Design review of the part built by this model. Coordinates are the model's own, in mm. Round coordinates to 2 decimals unless told otherwise and drop trailing zeros. Loops run counter-clockwise (first coordinate to the right, second up) from the corner with the lowest first, then second, coordinate; pieces in that order, holes last. Notation, with made-up numbers: (32.25, 40.5) - (53.25, 40.5) arc R6 ccw to (53.25, 51.5) - close; hole circle Ø11 at (61, 85.5). An arc over 180 degrees is marked (long way). Return JSON: item names as keys, results as strings. Group by question number.
from build123d import *

# Parameters (mm, degrees)
SKETCH1_R           = 92.075
SKETCH1_R_2         = 88.9
BOSS_EXTRUDE1_DEPTH = 38.1
SKETCH3_R           = 1.35255
CUT_EXTRUDE1_DEPTH  = 34.798
CIRPATTERN1_COUNT   = 3


with BuildPart() as part:
    # Sketch1 → Boss-Extrude1 (new, symmetric)
    with BuildSketch(Plane(origin=(0, 0, 0), x_dir=(1, 0, 0), z_dir=(0, 1, 0))):
        with Locations(Location((0, 0, 0), (0, 0, 90))):
            Circle(SKETCH1_R)
        with Locations(Location((0, 0, 0), (0, 0, 90))):
            Circle(SKETCH1_R_2, mode=Mode.SUBTRACT)
    extrude(amount=BOSS_EXTRUDE1_DEPTH, both=True)

    # Sketch3 → Cut-Extrude1 (cut)
    with BuildSketch(Plane(origin=(92.075, 0, 0), x_dir=(0, 0, -1), z_dir=(1, 0, 0))):
        with Locations((0, -31.75)):
            Circle(SKETCH3_R)
        with Locations((0, 31.75)):
            Circle(SKETCH3_R)
    cut_extrude1 = extrude(amount=-CUT_EXTRUDE1_DEPTH, mode=Mode.SUBTRACT)

    # CirPattern1: Cut-Extrude1 ×3 about axis
    cirpattern1_axis = Axis((0, 38.1, 0), (0, -1, 0))
    for i in range(1, CIRPATTERN1_COUNT):
        add(cut_extrude1.rotate(cirpattern1_axis, i * 360 / CIRPATTERN1_COUNT), mode=Mode.SUBTRACT)


solid = part.part
Q1. For line 1 (Y direction, x = 91, z = 0); line 2 (X direction, y = 5.5, z = 0) (3 decimals); line 3 (X direction, y = -28.5, z = 2.5), list the stretches that pass through material, from the lowest coordinate up.
Q2. Add section A-A, the plane z = -48. State the section outline as (x, y) points.
Q3. Draft analysis for pull direction X (two halves, no side actions). For faces 1 (the cylindrical face through (-74.96, -0.53, -47.79)), 2 (the cylindrical face through (89.885, 0.533, 19.96)), 3 (the flat face through (-48.2, 38.1, 75.5)), state which applies: pulls with the +X half, pulls with the -X half, needs draft (parallel to the pull), parting line crosses it, or undercut.
Q4. Add section C-C, the plane y = -24.5. State the section outline as (x, z) points (3 decimals).
Q5. Add section B-B, the plane x = -67.5. State the section outline as (y, z) points, plus the area to 3 significant figures.
Q6. Insertion check: pin 1 Ø8 at (y, z) = (8.5, 24.5) entering from +X; pin 2 Ø6 at (x, y) = (-13, 14) entering from -Z; pin 3 Ø1.5 at (x, y) = (21, 7.5) entering from +Z. Each pin has a flat end and moves straight along its axis. Give the tip position at first contact, or say it passes through.
Evaluation:
{
 "1": {"line 1": "-38.1 to -33.1, -30.4 to 30.4, 33.1 to 38.1", "line 2": "-92.075 to -88.9, 88.9 to 92.075", "line 3": "-92.04 to -88.86, 88.86 to 92.04"},
 "2": {"outline": "(-78.57, -38.1) - (-74.83, -38.1) - (-74.83, 38.1) - (-78.57, 38.1) - close; (74.83, -38.1) - (78.57, -38.1) - (78.57, 38.1) - (74.83, 38.1) - close"},
 "3": {"face 1": "undercut", "face 2": "parting line crosses it", "face 3": "needs draft"},
 "4": {"outline": "circle Ø184.15 at (0, 0); hole circle Ø177.8 at (0, 0)"},
 "5": {"outline": "(-38.1, -62.62) - (38.1, -62.62) - (38.1, -57.85) - (-38.1, -57.85) - close; (-38.1, 57.85) - (38.1, 57.85) - (38.1, 62.62) - (-38.1, 62.62) - close", "area": "727 mm²"},
 "6": {"pin 1": "x = 89.76", "pin 2": "z = -91.53", "pin 3": "z = 89.82"}
}
